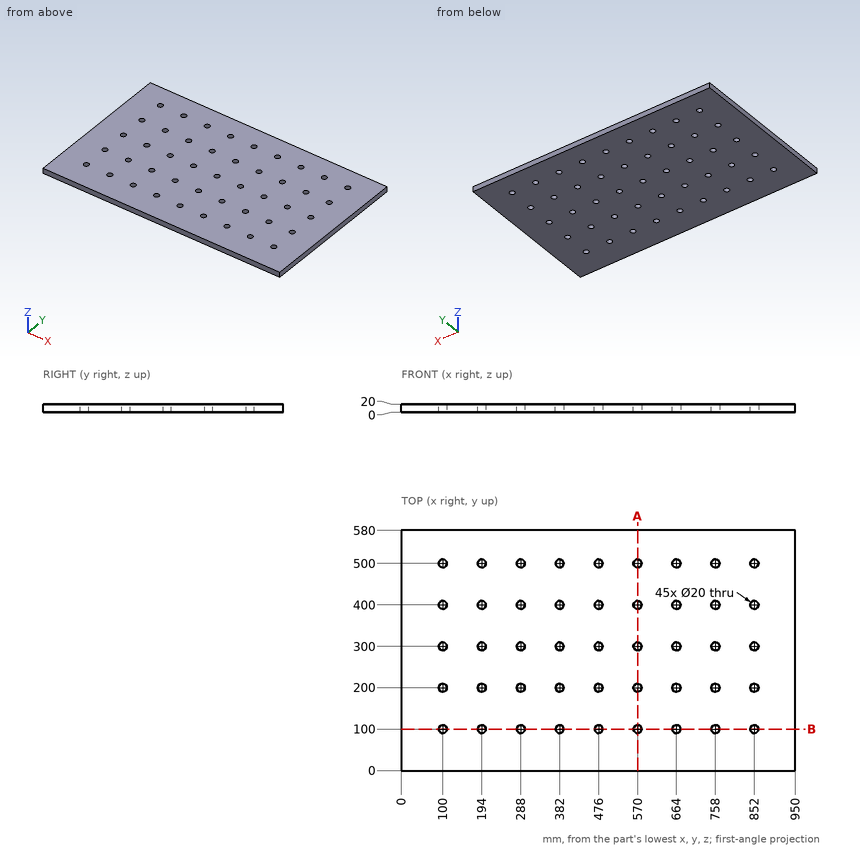
Drawing for the job (mm, zero at the part's lowest x, y, z). Coordinates: 2 decimals unless noted, no trailing zeros. Order: outer loops, then holes, each group sorted by start corner. A loop starts at its lowest first (then second) coordinate and runs counter-clockwise, first axis right, second up. Notation, with made-up numbers: (-24, 70) -> (-8, 70) arc R13 ccw to (-8, 85) -> close; hole circle Ø8 at (-4, 46.25). An arc over 180 degrees is marked (long way). Answer in a Markdown table with one row per item.
1) Band-saw the part on A-A (x = 570). List the corners of the cut face in (y, z), and give its area (3 significant figures).
Check values:
| item | result |
|---|---|
| outline | (0, 0) -> (90, 0) -> (90, 20) -> (0, 20) -> close; (110, 0) -> (190, 0) -> (190, 20) -> (110, 20) -> close; (210, 0) -> (290, 0) -> (290, 20) -> (210, 20) -> close; (310, 0) -> (390, 0) -> (390, 20) -> (310, 20) -> close; (410, 0) -> (490, 0) -> (490, 20) -> (410, 20) -> close; (510, 0) -> (580, 0) -> (580, 20) -> (510, 20) -> close |
| area | 9,600 mm2 |
2) Band-saw the part on B-B (y = 100). Give the number of separate pieces and of enclosed holes in the cut face, and give its area (3 significant figures).
Check values:
| item | result |
|---|---|
| separate pieces | 10 |
| enclosed holes | 0 |
| area | 15,400 mm2 |
3) Flat gauge pins, fed straight in: P1, Ø1, axis at x = 228.5, y = 96, coming from the -Z side; P2, Ø16, axis at x = 758, y = 100, coming from the -Z side (3 decimals). Where does each tip first touch, or does it go through?
Check values:
| item | result |
|---|---|
| P1 | z = 0 |
| P2 | through |
4) Drill centre lines: line 1 (Y direction, x = 381, z = 14.5); line 2 (Y direction, x = 852, z = 6). Where is each one in solid material? Low to high.
Check values:
| item | result |
|---|---|
| line 1 | 0 to 90.05, 109.95 to 190.05, 209.95 to 290.05, 309.95 to 390.05, 409.95 to 490.05, 509.95 to 580 |
| line 2 | 0 to 90, 110 to 190, 210 to 290, 310 to 390, 410 to 490, 510 to 580 |
